Could you check a few things on this model? Use its own coordinates, in mm. A direction names the side the tool comes from. Give positions to 0.01 mm unless a question says otherwise; leave off trailing zeros. Loops run counter-clockwise (first coordinate to the right, second up) from the corner with the lowest first, then second, coordinate; pieces in that order, holes last. Notation, with made-up numbers: (73.5, 36) -> (82.5, 36) arc R11 ccw to (82.5, 54) -> close; hole circle Ø5 at (7.5, -38). An arc over 180 degrees is marked (long way). Write item = value, one per line. Start each with the question number.
1) I need wall thicknesses on probe 1 along Z at (x, y) = (2.5, -3); probe 2 along Z at (x, y) = (0.25, 1.25); probe 3 along Y at (x, z) = (-1.5, -11.5). Which ranges of each line are inside material? Lowest first, please. Write a range as from..to.
2) I want a section at B-B (y = 0). List the corners of the cut face in (x, z) for me.
3) If we mould it in two halves opening along X, with no side actions, what happens to faces 1 (the face through (-1.261, 2.167, 2.414)), 2 (the face through (-0.54, -2.44, -24.4)), 3 (the face through (0, 0, -50))? For each: +X half, -X half, draft (parallel to the pull), parting line (faces both ways), or undercut.
4) I'm going to push flat-ended pins straight in: pin 1 Ø1.5 at (x, y) = (-2, 2) entering from -Z; pin 2 Ø1.5 at (x, z) = (3, -13.5) entering from -Y; pin 3 Ø5 at (y, z) = (3, -44) entering from -X. Where does each tip first touch, or does it pass through?
5) On a 3-axis mill with a long thin cutter (end or side, diameter ignored), from which of +Z, -Z, +X, -X, +Y, -Y can I reach the whole of each face in a straight line? I mean faces 4 (the face through (2, 2, 0)), 5 (the face through (1.2, 2.2, 2.4)), 6 (the face through (4.006, -1.262, 1.679)). Say none if no direction works.
6) I want a section at A-A (z = -28). List the corners of the cut face in (x, y) for me, and give its area (3 significant figures).
Autodesk Inventor part; units mm, degrees
ref_plane "YZ Plane" through (0, 0, 0) normal (1, 0, 0) x (0, 1, 0)
ref_plane "XZ Plane" through (0, 0, 0) normal (0, 1, 0) x (-1, 0, 0)
ref_plane "XY Plane" through (0, 0, 0) normal (0, 0, 1) x (1, 0, 0)
sketch "Sketch1" plane through (0, 0, 0) normal (0, 0, 1) x (1, 0, 0)
  circle A0 centre (0, 0) radius 4.2
  circle A1 centre (0, 0) radius 2.5
  dimension "d0" = 8.4
  dimension "d3" = 5
extrude "Extrusion1" add sketch "Sketch1" along normal blind 3.4 contours A0 | A1
extrude "Extrusion2" add sketch "Sketch1" against normal blind 50 contours A1
thread "Thread1"
fillet "Fillet1" radius 0.2 2 edges at (-4.2, 0, 3.4) (-4.2, 0, 0)
chamfer "Chamfer1" distance 0.5 angle 45 1 edges at (-2.5, 0, -50)
sketch "Sketch2" plane through (0, 0, 3.4) normal (0, 0, 1) x (1, 0, 0)
  line L0 (-2.5, 1.4593) -> (0.0138, 2.8947)
  line L1 (0.0138, 2.8947) -> (2.5138, 1.4354)
  line L2 (2.5138, 1.4354) -> (2.5, -1.4593)
  line L3 (2.5, -1.4593) -> (-0.0138, -2.8947)
  line L4 (-0.0138, -2.8947) -> (-2.5138, -1.4354)
  line L5 (-2.5138, -1.4354) -> (-2.5, 1.4593)
  point P0 (0, 0)
  point P1 (0, 0)
extrude "Extrusion3" cut sketch "Sketch2" against normal blind 2
properties part number "COTS_GENERIC_M5x50_Screw" material "Steel, Carbon"
Answer list:
q1.probe_1 = 0..3.4
q1.probe_2 = -50..1.4
q1.probe_3 = -2..2
q2.outline = (-4.2, 0.2) arc R0.2 ccw to (-4, 0) -> (-2.5, 0) -> (-2.5, -49.5) -> (-2, -50) -> (2, -50) -> (2.5, -49.5) -> (2.5, 0) -> (4, 0) arc R0.2 ccw to (4.2, 0.2) -> (4.2, 3.2) arc R0.2 ccw to (4, 3.4) -> (2.51, 3.4) -> (2.51, 1.4) -> (-2.51, 1.4) -> (-2.51, 3.4) -> (-4, 3.4) arc R0.2 ccw to (-4.2, 3.2) -> close
q3.face_1 = undercut
q3.face_2 = parting line
q3.face_3 = draft
q4.pin_1 = -49.92
q4.pin_2 = -1.09
q4.pin_3 = -2.45
q5.face_4 = -Z
q5.face_5 = +Z
q5.face_6 = +Z, -Z
q6.outline = circle Ø5 at (0, 0)
q6.area = 19.6 mm^2
